Part print with two shaded views. Sizes in mm from the minimum x, y, z corner. A direction names the side the tool comes from. Give positions to 0.01 mm unless a question says otherwise; leave off trailing zeros. Write each loop counter-clockwise with the first axis right and the second up, starting at its lowest first coordinate (ties: lowest second). Pieces come first, ordered by that corner, then holes. Notation, with made-up numbers: (-0.5, 12) - (31.5, 12) arc R17 cw to (31.5, 33) - close; hole circle Ø4 at (77.25, -39). An arc over 180 degrees is marked (long way). One line per item, written item: value. Start each with the question number.
(1) Drop flat-ended pins along their axis: P1, Ø8, axis at y = 8.5, z = 14.5, coming from the -X side; P2, Ø2, axis at x = 4, y = 15, coming from the -Z side; P3, Ø5, axis at y = 15.5, z = 32, coming from the -X side. Give the stop position or say it passes through.
(2) Cut at A-A, the plane x = 10. List the corners of the cut face in (y, z).
(3) 3-axis set-ups, long thin cutter, end or side, ignore diameter. For the marked faces 1 and 2: which of +Z, -Z, +X, -X, +Y, -Y reach the whole face in a straight line?
(4) Cut at C-C, the plane z = 9. List the corners of the cut face in (x, y), and give its area (3 significant figures).
(5) Probe L1, parallel to Z at x = 2.25, y = 13.5; L2, parallel to Y at x = 10.25, z = 23; L3, parallel to Y at x = 7, z = 17. List the from-to ranges inside material, lowest first.
(6) Cut at D-D, the plane z = 21. List the corners of the cut face in (x, y).
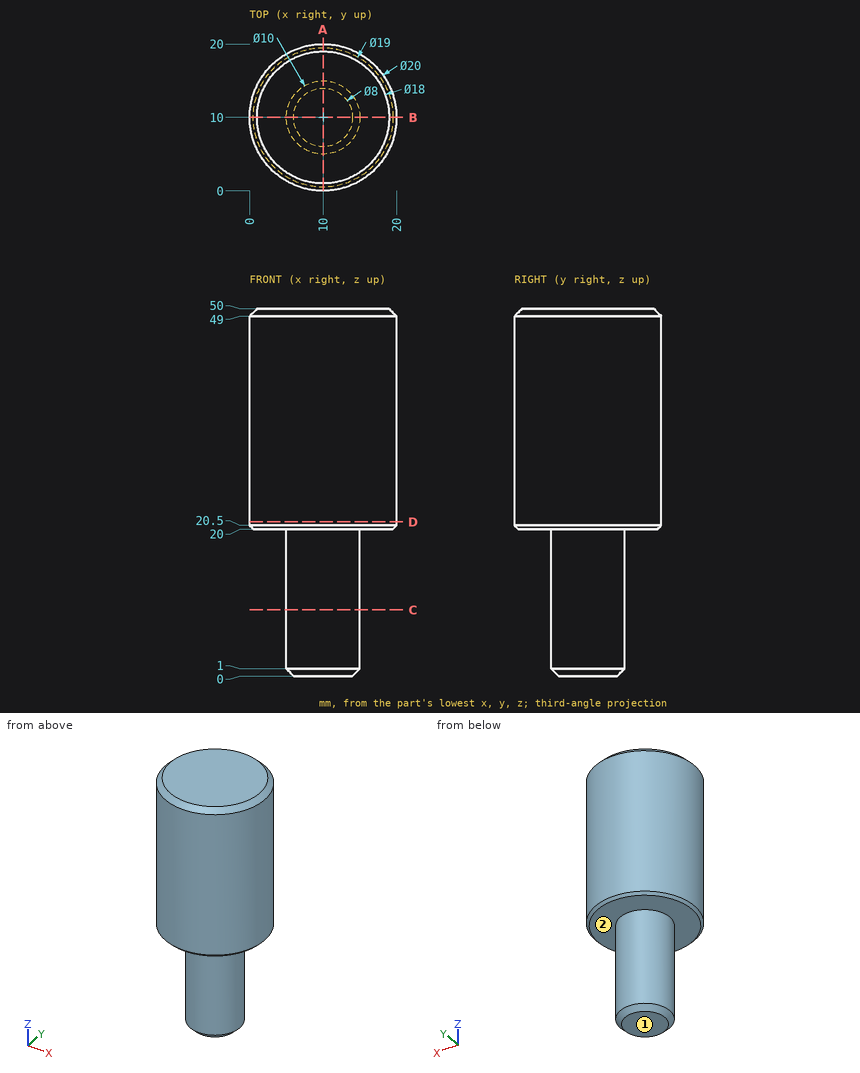
Answers follow:
1. P1: stops at x = 5
1. P2: stops at z = 20
1. P3: stops at x = 0.46
2. outline: (0, 20.5) - (0.5, 20) - (5, 20) - (5, 1) - (6, 0) - (14, 0) - (15, 1) - (15, 20) - (19.5, 20) - (20, 20.5) - (20, 49) - (19, 50) - (1, 50) - (0, 49) - close
3. face 1: -Z, +X, -X, +Y, -Y
3. face 2: -Z
4. outline: circle Ø10 at (10, 10)
4. area: 78.5 mm²
5. L1: z = 20 to 50
5. L2: y = 0 to 20
5. L3: y = 6 to 14
6. outline: circle Ø20 at (10, 10)
